Answer from the drawing. Dimensions are ordinates in mm from the lowest x, y and z of the part. Give positions to 0.01 mm unless a question says otherwise; leave off trailing zeros. Order: outer loops, then holes, each group sorted by start corner. A loop starts at its lowest first (then second) coordinate and runs counter-clockwise, first axis right, second up. Notation, with made-up numbers: (4.25, 19) -> (40.25, 19) arc R18 ccw to (40.25, 47) -> close; hole circle Ø5 at (-3.75, 53). An arc over 180 degrees is marked (long way). Answer as a JSON object with one key per item and string values. Group by question number.
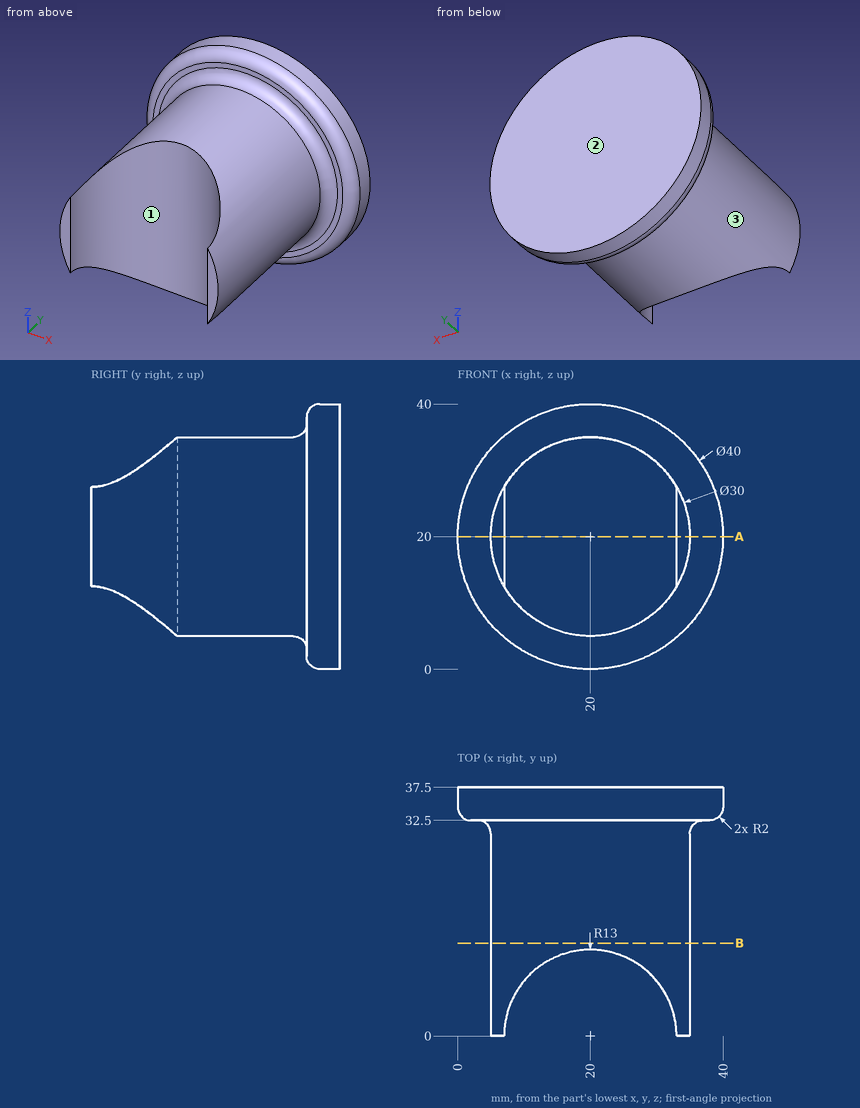
(1) Flat-ended cylindrical pins translate along their axes: pin 1 Ø3 at (y, z) = (9.5, 30.5) entering from +X; pin 2 Ø10 at (x, z) = (23.5, 13.5) entering from -Y; pin 3 Ø10 at (x, y) = (5.5, 18) entering from +Z. Find the tip coordinate at first contact, or state that the pin passes through.
(2) For a pull along X with two mould halves and no side action, classify the marked faces 1, 2 and 3 as +X half, -X half, draft (parallel to the pull), parting line (faces both ways), or undercut.
(3) A cutting plane is placed at A-A (z = 20). Determine the outline of the cut face in (x, y).
(4) Find the intervals of material crossed by line 1 along X through (y, z) = (12, 24); line 2 along Y through (x, z) = (28.5, 5.5); line 3 along X through (y, z) = (10, 15.5), in increasing order. Write a range as [from, to].
(5) A cutting plane is placed at B-B (y = 14). Determine the outline of the cut face in (x, z).
Check sheet entries:
{
 "1": {"pin 1": "stops at x = 32", "pin 2": "stops at y = 9.84", "pin 3": "stops at z = 31.61"},
 "2": {"face 1": "undercut", "face 2": "draft", "face 3": "parting line"},
 "3": {"outline": "(0, 34.5) arc R2 ccw to (2, 32.5) -> (3, 32.5) arc R2 cw to (5, 30.5) -> (5, 0) -> (7, 0) arc R13 cw to (33, 0) -> (35, 0) -> (35, 30.5) arc R2 cw to (37, 32.5) -> (38, 32.5) arc R2 ccw to (40, 34.5) -> (40, 37.5) -> (0, 37.5) -> close"},
 "4": {"line 1": "x = [5.54, 15], [25, 34.46]", "line 2": "y = [32.49, 37.5]", "line 3": "x = [5.69, 11.69], [28.31, 34.31]"},
 "5": {"outline": "circle Ø30 at (20, 20)"}
}
